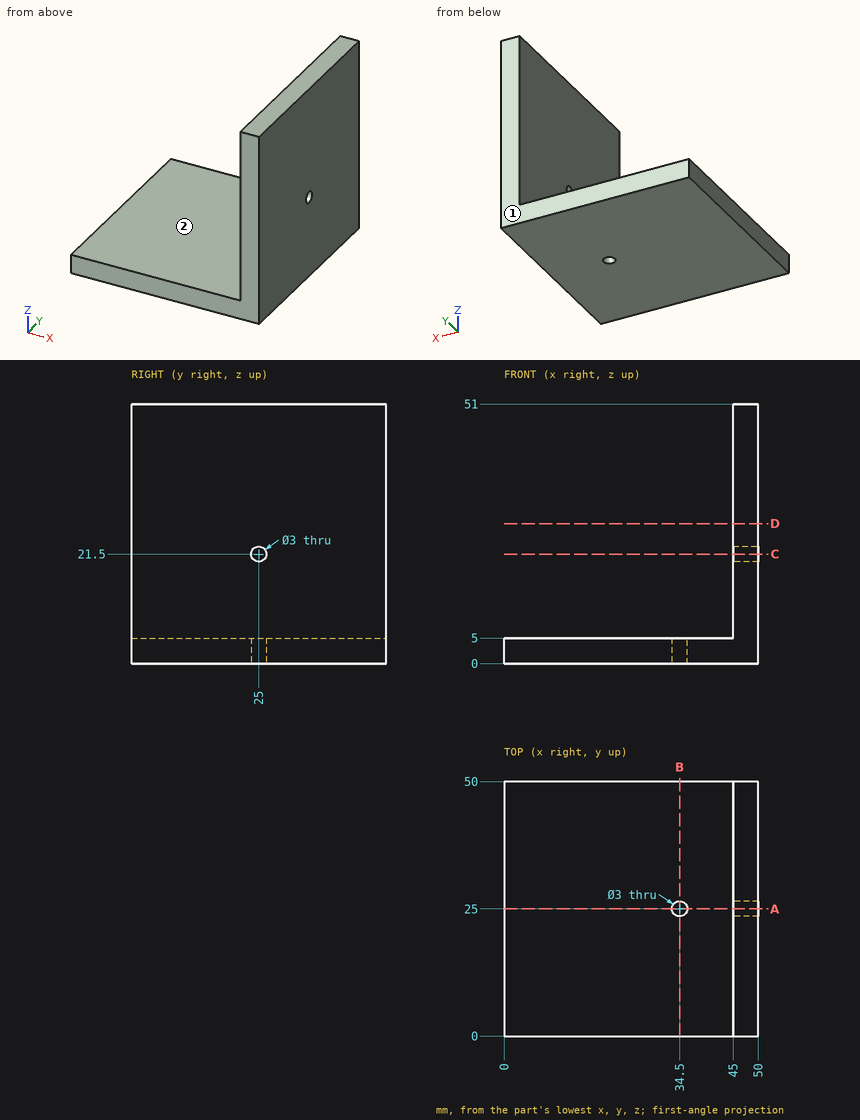
Could you check a few things on this drawing? It's one solid part, dimensions in mm from its lowest x, y, z. A direction names the side the tool comes from. Coordinates: 2 decimals unless noted, no trailing zeros. Loops run counter-clockwise (first coordinate to the right, second up) from the corner with the lowest first, then second, coordinate; pieces in that order, holes last.
1. For P1, Ø23, axis at y = 25, z = 30, coming from the -X side; P2, Ø1.8, axis at y = 25, z = 21.5, coming from the +X side; P3, Ø5, axis at x = 19.5, y = 28, coming from the +Z side, each with a flat end and sliding along its axis, tell me the tip position at first contact or that it passes through.
2. Imagine slicing it at B-B (x = 34.5). Please give me the cut outline in (y, z), and give its area (3 significant figures).
3. Imagine slicing it at A-A (y = 25). Please give me the cut outline in (x, z), and give its area (3 significant figures).
4. For the marked faces 1 and 2, which set-ups out of +Z, -Z, +X, -X, +Y, -Y let a thin tool reach every point of the face, with its end or its side?
5. I need wall thicknesses on L1, parallel to X at y = 25, z = 1.5; L2, parallel to X at y = 36, z = 46; L3, parallel to Z at x = 23, y = 28. Which ranges of each line are inside material? Lowest first, please.
6. Imagine slicing it at C-C (z = 21.5). Please give me the cut outline in (x, y), and give its area (3 significant figures).
7. Imagine slicing it at D-D (z = 27.5). Please give me the cut outline in (x, y), and give its area (3 significant figures).
Computed values:
1. P1: stops at x = 45
1. P2: passes through
1. P3: stops at z = 5
2. outline: (0, 0) - (23.5, 0) - (23.5, 5) - (0, 5) - close; (26.5, 0) - (50, 0) - (50, 5) - (26.5, 5) - close
2. area: 235 mm2
3. outline: (0, 0) - (33, 0) - (33, 5) - (0, 5) - close; (36, 0) - (50, 0) - (50, 20) - (45, 20) - (45, 5) - (36, 5) - close; (45, 23) - (50, 23) - (50, 51) - (45, 51) - close
3. area: 450 mm2
4. face 1: +Z, -Z, +X, -X, +Y
4. face 2: +Z, -X, +Y, -Y
5. L1: x = 0 to 33, 36 to 50
5. L2: x = 45 to 50
5. L3: z = 0 to 5
6. outline: (45, 0) - (50, 0) - (50, 23.5) - (45, 23.5) - close; (45, 26.5) - (50, 26.5) - (50, 50) - (45, 50) - close
6. area: 235 mm2
7. outline: (45, 0) - (50, 0) - (50, 50) - (45, 50) - close
7. area: 250 mm2
